Check sheet for the drawn part. Datum: minimum x, y, z corner. Units: mm. Round coordinates to 2 decimals unless told otherwise and drop trailing zeros. Write each loop counter-clockwise with the first axis right and the second up, starting at its lowest first coordinate (ties: lowest second). Pieces come first, ordered by that corner, then holes. Notation, with made-up numbers: M 30.25,44.25 L 51.25,44.25 A19 cw 51.25,49.25 Z; hole C -2.75,-26.5 d6. An arc over 180 degrees is marked long. One line per item, written item: value. Start each with the question number.
1. Section check D-D (x = 16). Record the boundary of the cut face in (y, z), and give its area (3 significant figures).
2. Section check A-A (x = 8). Record the boundary of the cut face in (y, z), and give its area (3 significant figures).
3. Scan lines: probe 1 along Z at (x, y) = (32, 4.8); probe 2 along Z at (x, y) = (8, 1.4); probe 3 along X at (y, z) = (2.35, 57). Record each from-to range of solid material in increasing order. Write a range as [from, to].
4. Section check B-B (z = 7). Record the boundary of the cut face in (x, y).
5. Depth check by flat-ended pin: P1, Ø1.8, axis at x = 16, z = 6, coming from the +Y side; P2, Ø5.5, axis at x = 16, z = 15, coming from the +Y side. Enter the tip coordinate at first touch or a pass-through.
6. Section check C-C (y = 4.9). Count the separate pieces of the cut face and the enclosed holes in it, and give its area (3 significant figures).
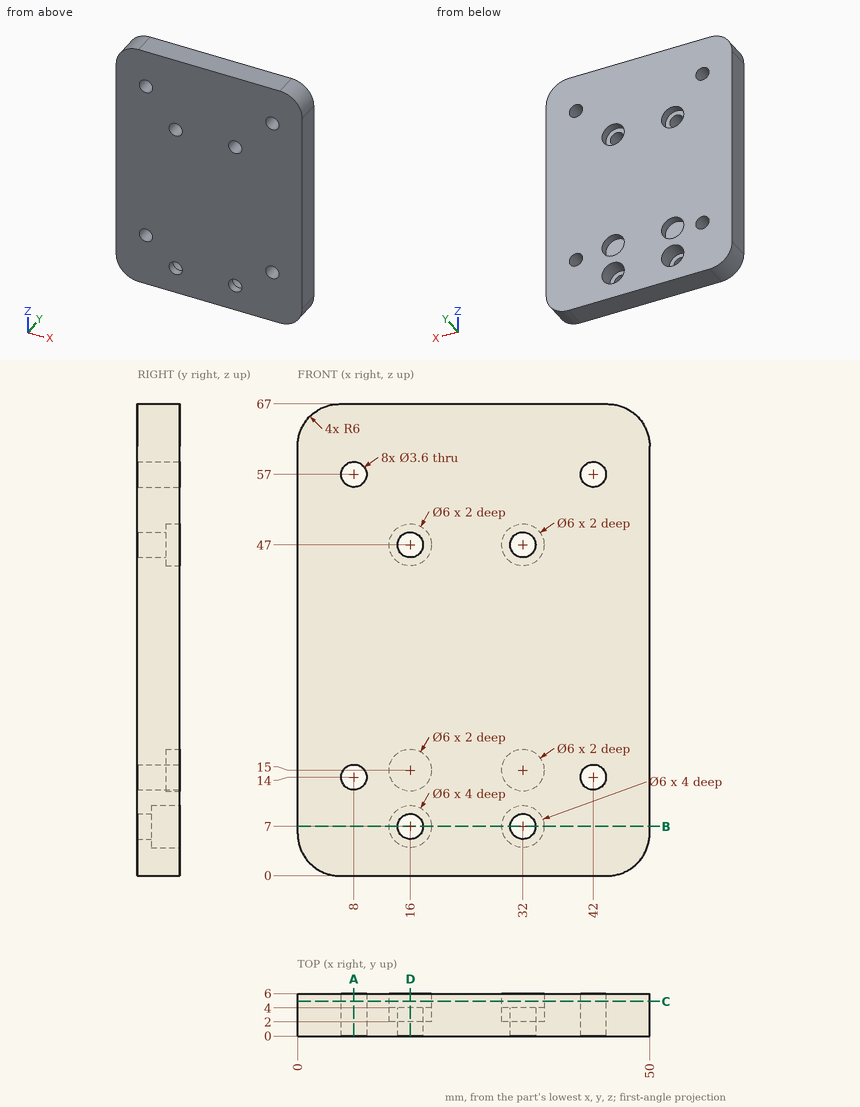
Result sheet:
1. outline: M 0,0 L 6,0 L 6,4 L 2,4 L 2,5.2 L 0,5.2 Z; M 0,8.8 L 2,8.8 L 2,10 L 6,10 L 6,12 L 4,12 L 4,18 L 6,18 L 6,44 L 4,44 L 4,45.2 L 0,45.2 Z; M 0,48.8 L 4,48.8 L 4,50 L 6,50 L 6,67 L 0,67 Z
1. area: 332 mm2
2. outline: M 0,0 L 6,0 L 6,12.2 L 0,12.2 Z; M 0,15.8 L 6,15.8 L 6,55.2 L 0,55.2 Z; M 0,58.8 L 6,58.8 L 6,67 L 0,67 Z
2. area: 359 mm2
3. probe 1: z = [0, 4], [10, 12], [18, 44], [50, 67]
3. probe 2: z = [0, 12.2], [15.8, 55.2], [58.8, 67]
3. probe 3: x = [0, 6.2], [9.8, 40.2], [43.8, 50]
4. outline: M 0,0 L 14.2,0 L 14.2,2 L 13,2 L 13,6 L 0,6 Z; M 17.8,0 L 30.2,0 L 30.2,2 L 29,2 L 29,6 L 19,6 L 19,2 L 17.8,2 Z; M 33.8,0 L 50,0 L 50,6 L 35,6 L 35,2 L 33.8,2 Z
5. P1: stops at y = 2
5. P2: stops at y = 4
6. separate pieces: 1
6. enclosed holes: 10
6. area: 3,110 mm2
